Design review of the part built by this model. Coordinates are the model's own, in mm. A direction names the side the tool comes from. Coordinates: 2 decimals unless noted, no trailing zeros. Loops run counter-clockwise (first coordinate to the right, second up) from the corner with the lowest first, then second, coordinate; pieces in that order, holes last. Notation, with made-up numbers: (41.25, 68) -> (54.25, 68) arc R23 ccw to (54.25, 76) -> close; hole circle Ø7 at (-18, -1). An arc over 180 degrees is marked (long way). Use one line per item in the form item = value. Start each with the question number.
1. Machinability: for faces 4 (the face through (1, -5, 2)), 5 (the face through (2, 3, 2)), which of the approach directions +Z, -Z, +X, -X, +Y, -Y give a long, thin tool a straight path to every point of the face, cutting with its end or side? Answer none if there is none.
2. Consider section C-C (z = 0). State the section outline as (x, y) points, then the cut area to 3 significant figures.
3. For pin 1 (1.5 mm diameter, centred on y = 2, z = 6.5, fed in from +X); pin 2 (6.5 mm diameter, centred on x = 0, z = 0, fed in from +Y), all flat-tipped, find the tip position at first contact; note any pin that passes through.
4. Consider section D-D (x = 85). State the section outline as (y, z) points.
5. Wall thickness on line 1 (X direction, y = -0.25, z = 0); line 2 (Z direction, x = 0, y = 4.5); line 3 (Z direction, x = 0, y = 1.5): over which ranges is each line inside the solid? List them lowest first. Write a range as from..to.
6. Consider section A-A (y = 0). State the section outline as (x, z) points, then the cut area to 3 significant figures.
7. The part is to be moulded in two halves that separate along X. For faces 1 (the face through (-98.246, 4.858, 8.319)), 2 (the face through (98.319, 4.858, 8.246)), 3 (the face through (-89.46, -0.07, -0.59)), say which applies: released by +X, released by -X, zero draft, split by the parting line, or undercut.
8. Consider section B-B (x = 0). State the section outline as (y, z) points, then the cut area to 3 significant figures.
Autodesk Inventor part; units mm, degrees
ref_plane "YZ Plane" through (0, 0, 0) normal (1, 0, 0) x (0, 1, 0)
ref_plane "XZ Plane" through (0, 0, 0) normal (0, 1, 0) x (-1, 0, 0)
ref_plane "XY Plane" through (0, 0, 0) normal (0, 0, 1) x (1, 0, 0)
sketch "Sketch1" plane through (0, 0, 0) normal (0, 1, 0) x (-1, 0, 0)
  line L0 (-100, 10) -> (100, 10)
  line L1 (100, 10) -> (100, -10)
  line L2 (100, -10) -> (-100, -10)
  line L3 (-100, -10) -> (-100, 10)
  line L4 (-100, 10) -> (100, -10) construction
  line L5 (100, 10) -> (-100, -10) construction
  point P0 (0, 0)
  dimension "Length" = 200
  dimension "Width" = 20
extrude "Extrusion1" add sketch "Sketch1" along normal mid plane 10
sketch "Sketch2" plane through (0, 5, 0) normal (0, 1, 0) x (1, 0, 0)
  circle A0 centre (0, 0) radius 2
  dimension "d4" = 4
extrude "Extrusion2" cut sketch "Sketch2" against normal up to surface (10 mm away)
sketch "Sketch3" plane through (0, 5, 0) normal (0, 1, 0) x (1, 0, 0)
  circle A0 centre (0, 0) radius 2
  point P0 (-15, 0)
  point P1 (15, 0)
  dimension "d7" = 30
  dimension "d8" = 15
hole "Hole1" [suppressed]
sketch "Sketch4" plane through (0, 5, 0) normal (0, 1, 0) x (1, 0, 0)
  point P0 (0, 0)
  point P1 (-85, 0)
  point P2 (85, 0)
  dimension "d16" = 170
  dimension "d17" = 85
hole "Hole2" at (-85, 5, 0) at (85, 5, 0) direction (0, -1, 0) diameter 9 end through all
sketch "Sketch5" plane through (0, 5, 0) normal (0, 1, 0) x (1, 0, 0)
  circle A0 centre (0, 0) radius 2
  circle A1 centre (0, 0) radius 3.5
  dimension "d25" = 7
extrude "Extrusion3" cut sketch "Sketch5" against normal blind 2
fillet "Fillet1" radius 5 4 edges at (-100, 0, 10) (-100, 0, -10) (100, 0, 10) (100, 0, -10)
chamfer "Chamfer1" distance 0.5 angle 45 8 edges at (0, 5, 10) (98.5355, 5, 8.5355) (100, 5, 0) (98.5355, 5, -8.5355) (0, 5, -10) (-98.5355, 5, -8.5355) (-100, 5, 0) (-98.5355, 5, 8.5355)
properties part number "Lower Arm Brass Plate" material "Brass, Soft Yellow"
Geometry check:
q1.face_4 = +Z, -Z, +X, -X, -Y
q1.face_5 = +Y
q2.outline = (-100, -5) -> (-89.5, -5) -> (-89.5, 5) -> (-99.5, 5) -> (-100, 4.5) -> close; (-80.5, -5) -> (-2, -5) -> (-2, 3) -> (-3.5, 3) -> (-3.5, 5) -> (-80.5, 5) -> close; (2, -5) -> (80.5, -5) -> (80.5, 5) -> (3.5, 5) -> (3.5, 3) -> (2, 3) -> close; (89.5, -5) -> (100, -5) -> (100, 4.5) -> (99.5, 5) -> (89.5, 5) -> close
q2.area = 1,770 mm²
q3.pin_1 = 99.94
q3.pin_2 = 3
q4.outline = (-5, -10) -> (4.5, -10) -> (5, -9.5) -> (5, -4.5) -> (-5, -4.5) -> close; (-5, 4.5) -> (5, 4.5) -> (5, 9.5) -> (4.5, 10) -> (-5, 10) -> close
q5.line_1 = -100..-89.5, -80.5..-2, 2..80.5, 89.5..100
q5.line_2 = -10..-3.5, 3.5..10
q5.line_3 = -10..-2, 2..10
q6.outline = (-100, -5) arc R5 ccw to (-95, -10) -> (95, -10) arc R5 ccw to (100, -5) -> (100, 5) arc R5 ccw to (95, 10) -> (-95, 10) arc R5 ccw to (-100, 5) -> close; hole circle Ø9 at (-85, 0); hole circle Ø4 at (0, 0); hole circle Ø9 at (85, 0)
q6.area = 3,840 mm²
q7.face_1 = released by -X
q7.face_2 = released by +X
q7.face_3 = undercut
q8.outline = (-5, -10) -> (4.5, -10) -> (5, -9.5) -> (5, -3.5) -> (3, -3.5) -> (3, -2) -> (-5, -2) -> close; (-5, 2) -> (3, 2) -> (3, 3.5) -> (5, 3.5) -> (5, 9.5) -> (4.5, 10) -> (-5, 10) -> close
q8.area = 154 mm²
